Answer from the drawing. Dimensions are ordinates in mm from the lowest x, y and z of the part. A direction names the side the tool comes from. Give positions to 0.01 mm unless a question says otherwise; leave off trailing zeros. Loops run counter-clockwise (first coordinate to the right, second up) from the corner with the lowest first, then second, coordinate; pieces in that order, holes last. Notation, with made-up numbers: (87.25, -38) -> (101.25, -38) arc R14 ccw to (101.25, -30) -> close; hole circle Ø6 at (56, 79.25). An arc over 180 degrees is marked (long way). Write each question's results on one line, items separated by ' | '. Start each with the question number.
Item 1: Section C-C on z = 11.5 is taken. Write down the section's boundary in (x, y) (1 decimal), and give its area (3 significant figures).
Item 2: Section A-A on x = 227 is taken. Write down the section's boundary in (y, z).
Item 3: Each of these flat-tipped pins is pushed along its axis until it touches: P1, Ø6, axis at y = 29, z = 90, coming from the +X side; P2, Ø3, axis at x = 287, z = 76, coming from the +Y side; P3, Ø3, axis at x = 287.5, z = 77.5, coming from the -Y side (1 decimal). Where does it stop, or does it pass through?
Item 4: Determine the mould class of the marked faces 1, 2 and 3 for opening direction Y: +Y half, -Y half, draft (parallel to the pull), parting line (faces both ways), or undercut.
Item 5: Which of the six approach directions +Z, -Z, +X, -X, +Y, -Y give full straight-line access (tool end or side, diameter ignored) to the marked faces 4 and 5?
Item 6: Section B-B on y = 127.5 is taken. Write down the section's boundary in (x, z) (1 decimal).
Item 7: Find the intervals of material crossed by line 1 (Y direction, x = 22, z = 136); line 2 (X direction, y = 82.5, z = 87.5) (1 decimal); line 3 (X direction, y = 36.5, z = 81) (1 decimal), in increasing order.
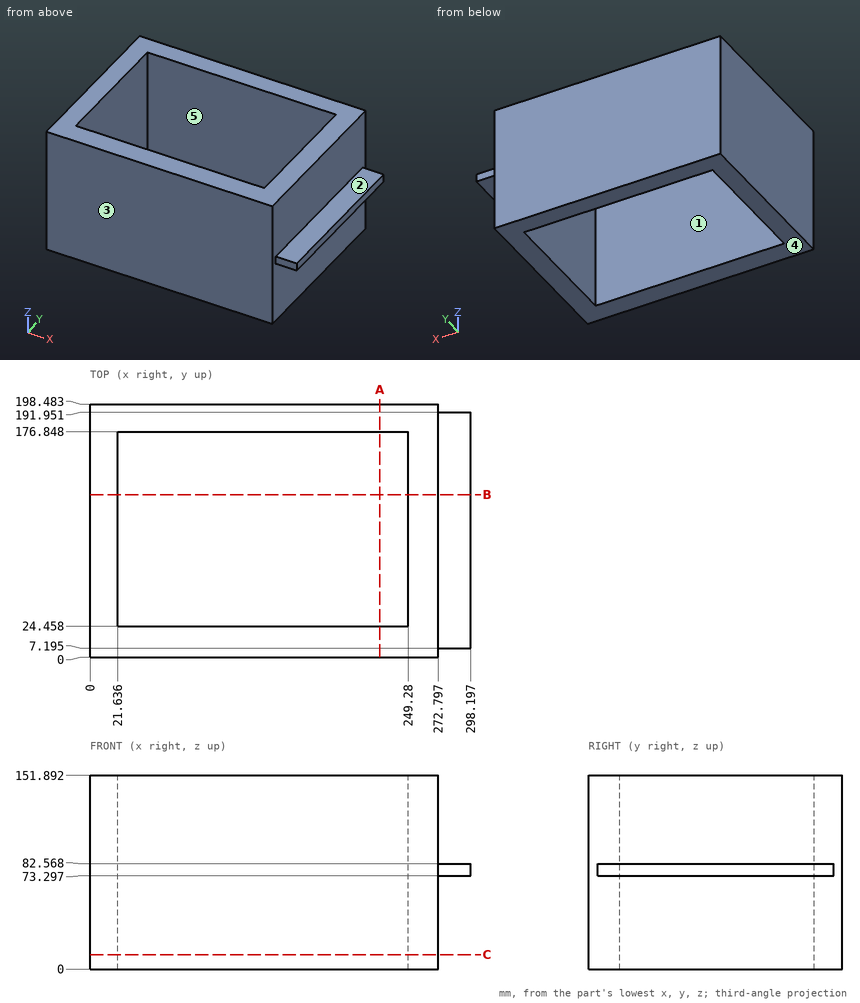
Findings:
1) outline: (0, 0) -> (272.8, 0) -> (272.8, 198.5) -> (0, 198.5) -> close; hole (21.6, 24.5) -> (249.3, 24.5) -> (249.3, 176.8) -> (21.6, 176.8) -> close | area: 19,500 mm2
2) outline: (0, 0) -> (24.46, 0) -> (24.46, 151.89) -> (0, 151.89) -> close; (176.85, 0) -> (198.48, 0) -> (198.48, 151.89) -> (176.85, 151.89) -> close
3) P1: x = 272.8 | P2: y = 191.95 | P3: y = 7.2
4) face 1: undercut | face 2: draft | face 3: -Y half
5) face 4: -Z, +X, -X, +Y, -Y | face 5: +Z, -Z
6) outline: (0, 0) -> (21.6, 0) -> (21.6, 151.9) -> (0, 151.9) -> close; (249.3, 0) -> (272.8, 0) -> (272.8, 73.3) -> (298.2, 73.3) -> (298.2, 82.6) -> (272.8, 82.6) -> (272.8, 151.9) -> (249.3, 151.9) -> close
7) line 1: 0 to 24.46, 176.85 to 198.48 | line 2: 0 to 21.6, 249.3 to 272.8 | line 3: 0 to 21.6, 249.3 to 298.2
